```python
from build123d import *

# Parameters (mm, degrees)
F1_DEPTH      = 2.5
F1_DEPTH_BACK = 2.5
F2_DEPTH      = 1.25
F2_DEPTH_BACK = 1.25


with BuildPart() as f1:
    # F0 (on Top) → F1 (new body, two sides)
    with BuildSketch(Plane.XY) as f1_sk:
        Polygon((0, 107), (0, 0), (82, 0), (80, 2), (2, 2), (2, 105), align=None)
        Polygon((6, 101), (2, 105), (2, 2), (80, 2), (76, 6), (6, 6), align=None)
    extrude(amount=F1_DEPTH)
    extrude(f1_sk.sketch, amount=-F1_DEPTH_BACK)

    # F0 (on Top) → F2 (cut, two sides)
    with BuildSketch(Plane.XY) as f2_sk:
        Polygon((6, 101), (2, 105), (2, 2), (80, 2), (76, 6), (6, 6), align=None)
    extrude(amount=-F2_DEPTH, mode=Mode.SUBTRACT)
    extrude(f2_sk.sketch, amount=F2_DEPTH_BACK, mode=Mode.SUBTRACT)


solid = f1.part
```
Model file for the job. Use its own axes, mm. A direction names the side the tool comes from. Coordinates: 2 decimals unless noted, no trailing zeros. Loops run counter-clockwise (first coordinate to the right, second up) from the corner with the lowest first, then second, coordinate; pieces in that order, holes last. Notation, with made-up numbers: M -36.75,38.25 L 8.25,38.25 A10 cw 8.25,54.25 Z; hole C -12.5,88.5 d1. An arc over 180 degrees is marked long. Use CSV: the item, a comma, the result in double quotes. Start each with the question number.
1. Flat gauge pins, fed straight in: pin 1 (2 mm diameter, centred on y = 65, z = -1.5, fed in from +X); pin 2 (0.8 mm diameter, centred on x = 52, z = 0.5, fed in from +Y); pin 3 (1 mm diameter, centred on x = 51.5, z = -2, fed in from +Y). Where does each tip first touch, or does it go through?
2. Tool access for faces 1 (the flat face through (3, 31, -1.25)), 2 (the flat face through (0, 54, 0)): list every direction of +Z, -Z, +X, -X, +Y, -Y with a clear straight run to the whole face (end or side of a thin tool).
3. Probe probe 1 along X at (y, z) = (9, -0.3); probe 2 along X at (y, z) = (80, -1.4). List the from-to ranges inside material, lowest first. Write a range as [from, to].
4. Band-saw the part on C-C, the plane z = -0.05. List the corners of the cut face in (x, y).
5. Band-saw the part on A-A, the plane x = 72.5. List the corners of the cut face in (y, z), then the cut area to 3 significant figures.
Entries:
1,pin 1,"stops at x = 6"
1,pin 2,"stops at y = 2"
1,pin 3,"stops at y = 6"
2,face 1,"+X, +Y"
2,face 2,"+Z, -Z, -X, +Y, -Y"
3,probe 1,"x = [0, 2]"
3,probe 2,"x = [0, 6]"
4,outline,"M 0,0 L 82,0 L 80,2 L 2,2 L 2,105 L 0,107 Z"
5,outline,"M 0,-2.5 L 6,-2.5 L 6,-1.25 L 2,-1.25 L 2,1.25 L 6,1.25 L 6,2.5 L 0,2.5 Z"
5,area,"20.0 mm2"
